Source: CAD feature listing. Evaluate the final solid. Frame: model axes, mm. Round coordinates to 2 decimals unless told otherwise and drop trailing zeros. Order: outer loops, then holes, each group sorted by start corner. A loop starts at its lowest first (then second) coordinate and runs counter-clockwise, first axis right, second up. Notation, with made-up numbers: (42, 84) - (54, 84) arc R19 ccw to (54, 115) - close; hole circle Ø1 at (7, -10.75). An arc over 180 degrees is marked (long way). Put each result on its own line as item: value. Start each with the question number.
1) Section D-D on x = 42.5. Output: boundary loops of the cut face in (y, z), then the cut area to 3 significant figures.
2) Section A-A on y = -16. Output: boundary loops of the cut face in (x, z).
3) Contact query for flat-ended pins moving along their axis: P1, Ø12, axis at x = 10, y = -11, coming from the +Z side; P2, Ø3, axis at y = -13, z = 3, coming from the -X side; P3, Ø2, axis at x = 18.5, z = 4, coming from the -Y side. Output: stop coordinate, or through.
4) Section B-B on x = 4. Output: boundary loops of the cut face in (y, z), then the cut area to 3 significant figures.
5) Section C-C on y = -5. Output: boundary loops of the cut face in (x, z).
6) Line query: probe 1 along Y at (x, z) = (42.5, 0.2); probe 2 along X at (y, z) = (-9, 2.7); probe 3 along X at (y, z) = (-7, 5.1). Output: solid intervals per line, ascending. Write a range as [from, to].
```python
from build123d import *

# Parameters (mm, degrees)
SKETCH_R        = 1.35
PAD_DEPTH       = 1
SKETCH002_W     = 4
SKETCH002_H     = 15
PAD001_DEPTH    = 5
POCKET_DEPTH    = 1.5
SKETCH004_W     = 34
SKETCH004_H     = 18
POCKET001_DEPTH = 5


with BuildPart() as part:
    # Sketch → Pad (new body)
    with BuildSketch(Plane.XY):
        with BuildLine():
            Line((-43.5, 20), (43.5, 20))
            ThreePointArc((46.5, 17), (45.62132, 19.12132), (43.5, 20))
            Line((46.5, 17), (46.5, -17))
            ThreePointArc((43.5, -20), (45.62132, -19.12132), (46.5, -17))
            Line((43.5, -20), (-43.5, -20))
            ThreePointArc((-46.5, -17), (-45.62132, -19.12132), (-43.5, -20))
            Line((-46.5, -17), (-46.5, 17))
            ThreePointArc((-43.5, 20), (-45.62132, 19.12132), (-46.5, 17))
        make_face()
        with Locations((-42.5, 16)):
            Circle(SKETCH_R, mode=Mode.SUBTRACT)
        with Locations((42.5, 16)):
            Circle(SKETCH_R, mode=Mode.SUBTRACT)
        with Locations((-42.5, -16)):
            Circle(SKETCH_R, mode=Mode.SUBTRACT)
        with Locations((42.5, -16)):
            Circle(SKETCH_R, mode=Mode.SUBTRACT)
    extrude(amount=PAD_DEPTH)

    # Sketch002 (on Face14 of Pad) → Pad001 (join)
    with BuildSketch(Plane.XY.offset(1)):
        with Locations((18.25, -10.5)):
            Rectangle(SKETCH002_W, SKETCH002_H)
        with Locations((-18.25, -10.5)):
            Rectangle(SKETCH002_W, SKETCH002_H)
    extrude(amount=PAD001_DEPTH)

    # Sketch003 (on Face21 of Pad001) → Pocket (cut)
    with BuildSketch(Plane(origin=(16.25, 0, 0), x_dir=(0, -1, 0), z_dir=(-1, 0, 0))):
        Polygon((3, 6), (3, 1), (17, 1), (17, 5), (7, 5), align=None)
    pocket = extrude(amount=-POCKET_DEPTH, mode=Mode.SUBTRACT)

    # Mirrored: Pocket across YZ
    add(pocket.mirror(Plane.YZ), mode=Mode.SUBTRACT)

    # Sketch004 (on Face5 of Mirrored) → Pocket001 (cut)
    with BuildSketch(Plane.XY.offset(1)):
        with Locations((0, 1)):
            Rectangle(SKETCH004_W, SKETCH004_H)
    extrude(amount=-POCKET001_DEPTH, mode=Mode.SUBTRACT)


solid = part.part
```
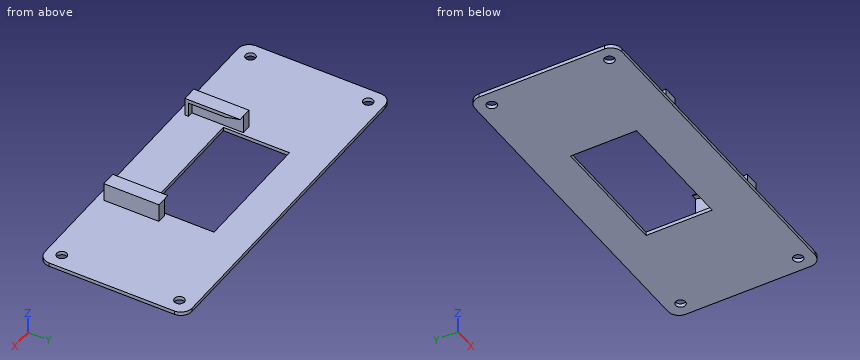
Answer sheet:
1. outline: (-20, 0) - (-17.35, 0) - (-17.35, 1) - (-20, 1) - close; (-14.65, 0) - (14.65, 0) - (14.65, 1) - (-14.65, 1) - close; (17.35, 0) - (20, 0) - (20, 1) - (17.35, 1) - close
1. area: 34.6 mm^2
2. outline: (-46.5, 0) - (-43.85, 0) - (-43.85, 1) - (-46.5, 1) - close; (-41.15, 0) - (41.15, 0) - (41.15, 1) - (20.25, 1) - (20.25, 6) - (16.25, 6) - (16.25, 5) - (17.75, 5) - (17.75, 1) - (-17.75, 1) - (-17.75, 5) - (-16.25, 5) - (-16.25, 6) - (-20.25, 6) - (-20.25, 1) - (-41.15, 1) - close; (43.85, 0) - (46.5, 0) - (46.5, 1) - (43.85, 1) - close
3. P1: z = 1
3. P2: x = -20.25
3. P3: y = -18
4. outline: (-20, 0) - (-8, 0) - (-8, 1) - (-20, 1) - close; (10, 0) - (20, 0) - (20, 1) - (10, 1) - close
4. area: 22.0 mm^2
5. outline: (-46.5, 0) - (-17, 0) - (-17, 1) - (-17.75, 1) - (-17.75, 5.5) - (-16.25, 5.5) - (-16.25, 6) - (-20.25, 6) - (-20.25, 1) - (-46.5, 1) - close; (16.25, 5.5) - (17.75, 5.5) - (17.75, 1) - (17, 1) - (17, 0) - (46.5, 0) - (46.5, 1) - (20.25, 1) - (20.25, 6) - (16.25, 6) - close
6. probe 1: [-20, -17.35], [-14.65, 14.65], [17.35, 20]
6. probe 2: [-20.25, -17.75], [17.75, 20.25]
6. probe 3: [-20.25, -16.25], [16.25, 20.25]
